Check sheet for the modelled part. Datum: model origin and axes. Units: mm. Face numbers are marked on the shaded views. A direction names the side the tool comes from. Round coordinates to 2 decimals unless told otherwise and drop trailing zeros. Order: outer loops, then holes, each group sorted by start corner. A loop starts at its lowest first (then second) coordinate and runs counter-clockwise, first axis right, second up. Notation, with made-up numbers: (-19, 58.5) -> (0, 58.5) arc R8 cw to (0, 64.5) -> close; hole circle Ø6 at (6, 74). An arc over 180 degrees is marked (long way). Answer in a Markdown table with one row per item. Add a question column.
1. Draft check along X on the marked faces 1 and 2. Enter one of: +X half, -X half, draft (parallel to the pull), parting line (faces both ways), or undercut.
2. Sectioned sample at B-B, the plane y = 1.25. Record the boundary of the cut face in (x, z), then the cut area to 3 significant figures.
3. Access from +Z, -Z, +X, -X, +Y, -Y to the whole of each face (thin tool, end or side, straight path). Record for the marked faces 3, 4, 5, 6 and 7.
4. Material ranges on L1, parallel to X at y = 7, z = -17.5; L2, parallel to Z at x = 21, y = 7; L3, parallel to Y at x = 13.5, z = -9, recorded low to high. Write a range as from..to.
5. Depth check by flat-ended pin: P1, Ø4.5, axis at y = 7, z = 12, coming from the -X side; P2, Ø2.5, axis at x = 12.5, z = 18, coming from the -Y side; P3, Ø1.5, axis at x = 63, z = 14.5, coming from the +Y side. Enter the tip coordinate at first touch or a pass-through.
6. Sectioned sample at A-A, the plane z = 11. Record the boundary of the cut face in (x, y), then the cut area to 3 significant figures.
7. Sectioned sample at C-C, the plane x = 63. Record the boundary of the cut face in (y, z), then the cut area to 3 significant figures.
8. Sectioned sample at D-D, the plane z = -12. Record the boundary of the cut face in (x, y).
Autodesk Inventor part; units mm, degrees
ref_plane "YZ Plane" through (0, 0, 0) normal (1, 0, 0) x (0, 1, 0)
ref_plane "XZ Plane" through (0, 0, 0) normal (0, 1, 0) x (-1, 0, 0)
ref_plane "XY Plane" through (0, 0, 0) normal (0, 0, 1) x (1, 0, 0)
sketch "Sketch1" plane through (0, 0, 0) normal (0, 0, 1) x (1, 0, 0)
  line L0 (0, 0) -> (2, 0)
  line L1 (2, 0) -> (2, 12.5)
  line L2 (2, 12.5) -> (0, 12.5)
  line L3 (0, 12.5) -> (0, 0)
  line L4 (2, 12.5) -> (6, 12.5)
  line L5 (6, 12.5) -> (6, 10.5)
  line L6 (6, 10.5) -> (2, 10.5)
  line L7 (2, 10.5) -> (2, 12.5)
  line L8 (6, 10.5) -> (4, 10.5)
  line L9 (4, 10.5) -> (4, 6.5)
  line L10 (4, 6.5) -> (6, 6.5)
  line L11 (6, 6.5) -> (6, 10.5)
  dimension "d0" = 2
  dimension "d1" = 12.5
  dimension "d2" = 4
  dimension "d3" = 2
  dimension "d4" = 2
  dimension "d5" = 4
extrude "Extrusion1" add sketch "Sketch1" along normal blind 5
sketch "Sketch2" plane through (6, 6.5, 0) normal (1, 0, 0) x (0, 0, -1)
  line L0 (-5, 4) -> (-5, 0)
  line L1 (0, 0) -> (0, 4)
  line L2 (-5, 0) -> (0, 0)
  line L3 (0, 0) -> (0, 2)
  line L4 (0, 2) -> (-5, 2)
  line L5 (-5, 2) -> (-5, 0)
  point P0 (0, -6.5)
  dimension "d8" = 2
extrude "Extrusion2" add sketch "Sketch2" along normal blind 10
sketch "Sketch3" plane through (0, 0, 0) normal (0, 0, -1) x (-1, 0, 0)
  line L0 (-16, 6.5) -> (-4, 6.5)
  line L1 (-16, 8.5) -> (-16, 6.5)
  line L2 (-16, 8.5) -> (-11, 8.5)
  line L3 (-11, 8.5) -> (-11, 6.5)
  line L4 (-11, 6.5) -> (-16, 6.5)
  line L5 (-16, 6.5) -> (-16, 8.5)
extrude "Extrusion3" add sketch "Sketch3" along normal blind 30
sketch "Sketch4" plane through (16, 6.5, 0) normal (1, 0, 0) x (0, 0, -1)
  line L0 (-5, 0) -> (30, 0)
  line L1 (30, 0) -> (30, 2)
  line L2 (30, 2) -> (25, 2)
  line L3 (25, 2) -> (25, 0)
  line L4 (25, 0) -> (30, 0)
  line L5 (30, 0) -> (30, 2)
  point P0 (0, -6.5)
  dimension "d13" = 5
extrude "Extrusion4" add sketch "Sketch4" along normal blind 50
sketch "Sketch5" plane through (16, 6.5, -25) normal (0, 0, 1) x (1, 0, 0)
  line L0 (-5, 0) -> (50, 0)
  line L1 (50, 2) -> (45, 2)
  line L2 (45, 2) -> (45, 0)
  line L3 (45, 0) -> (50, 0)
  line L4 (50, 0) -> (50, 2)
  point P0 (-16, -6.5)
  dimension "d16" = 5
extrude "Extrusion5" add sketch "Sketch5" along normal blind 30
sketch "Sketch6" plane through (66, 6.5, 0) normal (1, 0, 0) x (0, 0, -1)
  line L0 (0, 0) -> (-5, 0)
  line L1 (-5, 2) -> (0, 2)
  line L2 (0, 2) -> (0, 0)
  line L3 (0, 0) -> (-5, 0)
  line L4 (-5, 0) -> (-5, 2)
  point P0 (0, -6.5)
extrude "Extrusion6" add sketch "Sketch6" along normal blind 29.93
sketch "Sketch7" plane through (95.93, 6.5, 0) normal (1, 0, 0) x (0, 0, -1)
  line L0 (0, 0) -> (0, 2)
  line L1 (0, 2) -> (-5, 2)
  line L2 (-5, 2) -> (-5, 0)
  line L3 (-5, 0) -> (0, 0)
  point P0 (0, -6.5)
extrude "Extrusion7" add sketch "Sketch7" along normal blind 4
sketch "Sketch8" plane through (4, 6.5, 0) normal (0, -1, 0) x (1, 0, 0)
  line L0 (62, 0) -> (95.93, 0)
  line L1 (57, 5) -> (95.93, 5)
  line L2 (95.93, 5) -> (93.93, 5)
  line L3 (93.93, 5) -> (93.93, 0)
  line L4 (93.93, 0) -> (95.93, 0)
  line L5 (95.93, 0) -> (95.93, 5)
  point P0 (-4, 0)
  dimension "d23" = 2
extrude "Extrusion8" add sketch "Sketch8" along normal blind 10
sketch "Sketch9" plane through (4, 6.5, 0) normal (0, -1, 0) x (1, 0, 0)
  line L0 (57, 5) -> (95.93, 5)
  line L1 (62, 0) -> (95.93, 0)
  line L2 (57, 5) -> (62, 5)
  line L3 (62, 5) -> (62, 0)
  line L4 (62, 0) -> (57, 0)
  line L5 (57, 0) -> (57, 5)
  line L6 (12, 5) -> (7, 5)
  line L7 (7, 5) -> (7, 0)
  line L8 (7, 0) -> (12, 0)
  line L9 (12, 0) -> (12, 5)
  line L10 (7, 5) -> (12, 5)
  line L11 (12, 5) -> (12, 0)
  line L12 (12, 0) -> (7, 0)
  line L13 (7, 0) -> (7, 5)
  line L14 (57, 5) -> (62, 5)
  line L15 (62, 5) -> (62, 0)
  line L16 (62, 0) -> (57, 0)
  line L17 (57, 0) -> (57, 5)
  point P0 (-4, 0)
extrude "Extrusion9" add sketch "Sketch9" along normal blind 2
sketch "Sketch10" plane through (0, 0, 5) normal (0, 0, 1) x (1, 0, 0)
  line L0 (16, 8.5) -> (16, 4.5)
  line L1 (11, 4.5) -> (16, 4.5)
  line L2 (16, 4.5) -> (16, 6.4)
  line L3 (16, 6.4) -> (11, 6.4)
  line L4 (11, 6.4) -> (11, 4.5)
  dimension "d28" = 1.9
extrude "Extrusion10" add sketch "Sketch10" along normal blind 20
sketch "Sketch11" plane through (16, 6.5, 5) normal (0, 0, 1) x (1, 0, 0)
  line L0 (50, 0) -> (50, -2)
  line L1 (45, -2) -> (50, -2)
  line L2 (50, -2) -> (50, -0.1)
  line L3 (50, -0.1) -> (45, -0.1)
  line L4 (45, -0.1) -> (45, -2)
  point P0 (-16, -6.5)
  dimension "d31" = 1.9
extrude "Extrusion11" add sketch "Sketch11" along normal blind 20
sketch "Sketch12" plane through (61, 6.5, -25) normal (-1, 0, 0) x (0, 0, 1)
  line L0 (0, 0) -> (25, 0)
  line L1 (30, 2) -> (30, -0.1)
  line L2 (0, 2) -> (30, 2)
  line L3 (12, 2) -> (18, 2)
  line L4 (18, 2) -> (18, 0)
  line L5 (18, 0) -> (12, 0)
  line L6 (12, 0) -> (12, 2)
  point P0 (25, -6.5)
  dimension "d34" = 6
  dimension "d35" = 12
extrude "Extrusion12" add sketch "Sketch12" along normal up to next
properties part number "Steunbalk boven bocht"
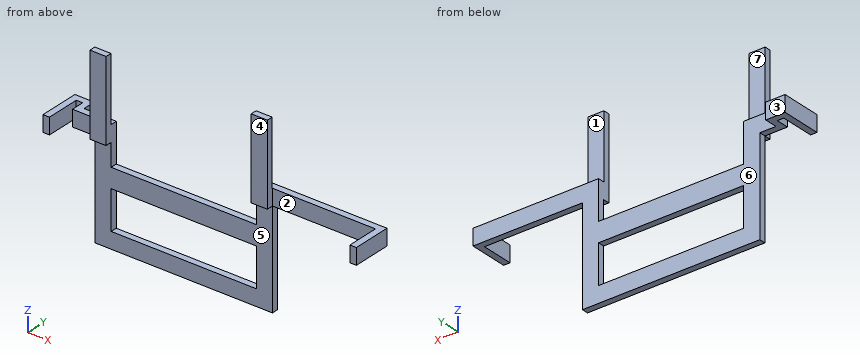
Answer key:
| question | item | result |
|---|---|---|
| 1 | face 1 | draft |
| 1 | face 2 | undercut |
| 2 | outline | (0, 0) -> (2, 0) -> (2, 5) -> (0, 5) -> close; (97.93, 0) -> (99.93, 0) -> (99.93, 5) -> (97.93, 5) -> close |
| 2 | area | 20.0 mm² |
| 3 | face 3 | +Z, -Z, +X, -X, +Y |
| 3 | face 4 | +Z, -Z, -Y |
| 3 | face 5 | -Z, +X, -X, -Y |
| 3 | face 6 | +Z, -Z, +X, +Y |
| 3 | face 7 | +Z, +X, -X, +Y |
| 4 | L1 | x = 11..16, 61..66 |
| 4 | L2 | z = -30..-25, -13..-7 |
| 4 | L3 | y = 6.5..8.5 |
| 5 | P1 | stops at x = 11 |
| 5 | P2 | stops at y = 4.5 |
| 5 | P3 | stops at y = 6.4 |
| 6 | outline | (11, 4.5) -> (16, 4.5) -> (16, 6.4) -> (11, 6.4) -> close; (61, 4.5) -> (66, 4.5) -> (66, 6.4) -> (61, 6.4) -> close |
| 6 | area | 19.0 mm² |
| 7 | outline | (4.5, 0) -> (6.5, 0) -> (6.5, -30) -> (8.5, -30) -> (8.5, 5) -> (6.4, 5) -> (6.4, 25) -> (4.5, 25) -> close |
| 7 | area | 118 mm² |
| 8 | outline | (11, 6.5) -> (66, 6.5) -> (66, 8.5) -> (11, 8.5) -> close |
